```python
from build123d import *

# Parameters (mm, degrees)
F0_R     = 12.5
F0_R_2   = 9.5
F1_DEPTH = 105
F2_R     = 12.5
F3_DEPTH = 3
F5_D     = 3.3
F5_DEPTH = 22.1
F5_TIP   = 0.9914200214
F7_D     = 4.4
F7_DEPTH = 22.1
F7_TIP   = 1.3218933619


with BuildPart() as f1:
    # F0 (on Top) → F1 (new body)
    with BuildSketch(Plane.XY):
        Circle(F0_R)
        Circle(F0_R_2, mode=Mode.SUBTRACT)
    extrude(amount=F1_DEPTH)

    # F2 (on face) → F3 (join)
    with BuildSketch(Plane.XY.offset(105)):
        Circle(F2_R)
    extrude(amount=-F3_DEPTH)

    # F5 (one way)
    with BuildSketch(Plane.XZ):
        with Locations((0, 12)):
            Circle(F5_D / 2)
    extrude(amount=-F5_DEPTH, mode=Mode.SUBTRACT)
    with Locations(Plane.XZ):
        with Locations((0, 12)):
            with Locations((0, 0, -(F5_DEPTH + F5_TIP / 2))):  # 118° drill point
                Cone(0, F5_D / 2, F5_TIP, mode=Mode.SUBTRACT)

    # F7 (one way)
    with BuildSketch(Plane(origin=(0, 0, 0), x_dir=(0, 1, 0), z_dir=(-1, 0, 0))):
        with Locations((0, -81), (0, -29)):
            Circle(F7_D / 2)
    extrude(amount=-F7_DEPTH, mode=Mode.SUBTRACT)
    with Locations(Plane(origin=(0, 0, 0), x_dir=(0, 1, 0), z_dir=(-1, 0, 0))):
        with Locations((0, -81), (0, -29)):
            with Locations((0, 0, -(F7_DEPTH + F7_TIP / 2))):  # 118° drill point
                Cone(0, F7_D / 2, F7_TIP, mode=Mode.SUBTRACT)


solid = f1.part
```
Input: part model. Units: mm. Frame: model coordinates. A direction names the side the tool comes from. Give positions to 0.01 mm unless a question says otherwise; leave off trailing zeros. Loops run counter-clockwise (first coordinate to the right, second up) from the corner with the lowest first, then second, coordinate; pieces in that order, holes last. Notation, with made-up numbers: M 30,52.5 L 59,52.5 A14 ccw 59,65.5 Z; hole C -36,6.25 d8. An arc over 180 degrees is marked long. Answer as CSV lines item,"result". Start each with the question number.
1. Section A-A on x = 0. Return loops of the section in (y, z).
2. Line query: L1, parallel to Z at x = 11.8, y = 0; L2, parallel to Y at x = 0, z = 66; L3, parallel to Z at x = -6.5, y = -3.75. Output: solid intervals per line, ascending.
3. Section B-B on y = 0. Return loops of the section in (x, z).
4. Pull-direction query (Z, two-part tool) for faces 4 (the face through (0, 0, 102)), 5 (the face through (0, 0, 105)), 6 (the face through (-0.4, 10.9, 10.4)); classes: released by +Z, released by -Z, zero draft, split by the parting line, or undercut.
5. Section D-D on x = -8.25. Return loops of the section in (y, z).
6. Section C-C on z = 72. Return loops of the section in (x, y), plus the area to 3 significant figures.
7. Pin query (flat end, axial travel): P1, Ø2, axis at x = 0, z = 12, coming from the +Y side; P2, Ø9.5, axis at x = -2, y = 1.5, coming from the -Z side; P3, Ø5, axis at y = -4, z = 16.5, coming from the +X side. Return the tip coordinate at first contact, or that it passes through.
8. Reachability of faces 1 (the face through (4.38, -8.43, 50.29)), 2 (the face through (10.848, -2.198, 28.903)), 3 (the face through (2.7, 9.3, 0)) from +Z, -Z, +X, -X, +Y, -Y: full face, straight path, thin tool, end or side. Return the list, or none.
Computed values:
1,outline,"M -12.5,0 L -9.5,0 L -9.5,102 L 9.5,102 L 9.5,13.65 L 12.5,13.65 L 12.5,105 L -12.5,105 Z; M 9.5,0 L 12.5,0 L 12.5,10.35 L 9.5,10.35 Z"
2,L1,"z = 0 to 26.8, 31.2 to 78.8, 83.2 to 105"
2,L2,"y = -12.5 to -9.5, 9.5 to 12.5"
2,L3,"z = 102 to 105"
3,outline,"M -12.5,0 L -9.5,0 L -9.5,102 L 9.5,102 L 9.5,83.2 L 12.5,83.2 L 12.5,105 L -12.5,105 Z; M 9.5,0 L 12.5,0 L 12.5,26.8 L 9.5,26.8 Z; M 9.5,31.2 L 12.5,31.2 L 12.5,78.8 L 9.5,78.8 Z"
4,face 4,"released by -Z"
4,face 5,"released by +Z"
4,face 6,"undercut"
5,outline,"M -9.39,0 L -4.71,0 L -4.71,102 L 4.71,102 L 4.71,0 L 9.39,0 L 9.39,105 L -9.39,105 Z"
6,outline,"C 0,0 d25; hole C 0,0 d19"
6,area,"207 mm²"
7,P1,"stops at y = -9.45"
7,P2,"stops at z = 102"
7,P3,"stops at x = 12.41"
8,face 1,"-Z"
8,face 2,"+X"
8,face 3,"-Z, +X, -X, +Y, -Y"
